Autodesk Inventor part; units mm, degrees
ref_plane "YZ Plane" through (0, 0, 0) normal (1, 0, 0) x (0, 1, 0)
ref_plane "XZ Plane" through (0, 0, 0) normal (0, 1, 0) x (-1, 0, 0)
ref_plane "XY Plane" through (0, 0, 0) normal (0, 0, 1) x (1, 0, 0)
sketch "Sketch1" plane through (0, 0, 0) normal (0, 0, 1) x (1, 0, 0)
  line L0 (-14.25, -14.5) -> (13.65, -14.5)
  line L1 (-13.65, -55.2958) -> (14.25, -55.2958)
  line L2 (50, 0) -> (-50, 0)
  line L3 (-50, 0) -> (-50, -90)
  line L4 (-50, -90) -> (50, -90)
  line L5 (50, -90) -> (50, 0)
  line L6 (50, -86.2958) -> (-50, -86.2958)
  line L7 (14.65, -6.65) -> (-15.25, -6.65)
  line L8 (-15.25, -6.65) -> (-15.25, -22.35)
  line L9 (-15.25, -22.35) -> (14.65, -22.35)
  line L10 (14.65, -22.35) -> (14.65, -6.65)
  line L11 (15.25, -47.4458) -> (-14.65, -47.4458)
  line L12 (-14.65, -47.4458) -> (-14.65, -63.1458)
  line L13 (-14.65, -63.1458) -> (15.25, -63.1458)
  line L14 (15.25, -63.1458) -> (15.25, -47.4458)
  line L15 (30.5, -65.2958) -> (29.35, -65.2958)
  line L16 (-30.5, -65.2958) -> (-29.35, -65.2958)
  circle A0 centre (20.65, -24.0677) radius 2.25
  circle A1 centre (22.6692, -56.1259) radius 2.25
  circle A2 centre (22.25, -13.4966) radius 2.25
  line L17 (19.75, -61.0677) -> (19.75, -50.9236)
  line L18 (19.75, -50.9236) -> (23.15, -50.9236)
  line L19 (23.15, -50.9236) -> (23.15, -46.7261)
  line L20 (19.75, -46.7261) -> (23.15, -46.7261)
  line L21 (19.75, -46.7261) -> (19.75, -44.8549)
  line L22 (19.75, -44.8549) -> (17.65, -44.8549)
  line L23 (17.65, 0) -> (17.65, -44.8549)
  line L24 (17.65, 0) -> (26.85, 0)
  line L25 (26.85, -65.2958) -> (26.85, 0)
  line L26 (23.15, -65.2958) -> (26.85, -65.2958)
  line L27 (23.15, -65.2958) -> (23.15, -61.0677)
  line L28 (19.75, -61.0677) -> (23.15, -61.0677)
  circle A3 centre (-24.3428, -2.5072) radius 2.25
  circle A4 centre (-20.65, -57.8419) radius 2.25
  circle A5 centre (-20.65, -44.9257) radius 2.25
  circle A6 centre (-23.3, -12.9282) radius 2.25
  line L29 (-26.85, 0) -> (-17.65, 0)
  line L30 (-17.65, -4.0591) -> (-17.65, 0)
  line L31 (-19.75, -4.0591) -> (-17.65, -4.0591)
  line L32 (-19.75, -4.7124) -> (-19.75, -4.0591)
  line L33 (-19.75, -4.7124) -> (-23.15, -4.7124)
  line L34 (-23.15, -4.7124) -> (-23.15, -8.7282)
  line L35 (-19.75, -8.7282) -> (-23.15, -8.7282)
  line L36 (-19.75, -18.8723) -> (-19.75, -8.7282)
  line L37 (-19.75, -18.8723) -> (-23.15, -18.8723)
  line L38 (-23.15, -18.8723) -> (-23.15, -23.0697)
  line L39 (-19.75, -23.0697) -> (-23.15, -23.0697)
  line L40 (-19.75, -24.9409) -> (-19.75, -23.0697)
  line L41 (-19.75, -24.9409) -> (-17.65, -24.9409)
  line L42 (-17.65, -65.2958) -> (-17.65, -24.9409)
  line L43 (-26.85, -65.2958) -> (-17.65, -65.2958)
  line L44 (-26.85, 0) -> (-26.85, -65.2958)
  line L45 (-17.65, -4.0591) -> (-17.65, -24.9409)
  line L46 (23.15, -65.2958) -> (17.65, -65.2958)
  line L47 (17.65, -65.2958) -> (17.65, -44.8549)
  line L48 (17.65, -6.65) -> (-17.65, -6.65)
  line L49 (-17.65, -63.1458) -> (17.65, -63.1458)
  line L50 (-26.85, -65.2958) -> (-26.85, -13)
  line L51 (-26.85, -65.2958) -> (-29.35, -65.2958)
  line L52 (-29.35, -65.2958) -> (-29.35, -19)
  line L53 (-29.35, -19) -> (-36.25, -19)
  line L54 (-36.25, -13) -> (-36.25, -19)
  line L55 (-26.85, -13) -> (-36.25, -13)
  line L56 (26.85, -13) -> (26.85, -65.2958)
  line L57 (26.85, -13) -> (36.25, -13)
  line L58 (36.25, -19) -> (36.25, -13)
  line L59 (29.35, -19) -> (36.25, -19)
  line L60 (29.35, -19) -> (29.35, -65.2958)
  line L61 (29.35, -65.2958) -> (26.85, -65.2958)
  line L62 (-26.85, -3) -> (-26.85, 0)
  line L63 (-26.85, -3) -> (-36.25, -3)
  line L64 (-36.25, 0) -> (-36.25, -3)
  line L65 (-26.85, 0) -> (-36.25, 0)
  line L66 (26.85, 0) -> (26.85, -3)
  line L67 (26.85, 0) -> (36.25, 0)
  line L68 (36.25, -3) -> (36.25, 0)
  line L69 (26.85, -3) -> (36.25, -3)
  arc A7 (26.85, -66.2958) -> (29.85, -69.2958) centre (29.85, -66.2958) ccw
  line L70 (26.85, -65.2958) -> (26.85, -66.2958)
  line L71 (26.85, -65.2958) -> (50, -65.2958)
  line L72 (50, -65.2958) -> (50, -85.9433)
  line L73 (34.5, -85.9433) -> (50, -85.9433)
  line L74 (34.5, -78.442) -> (34.5, -85.9433)
  line L75 (34.5, -78.442) -> (45.421, -78.442)
  arc A8 (45.421, -78.442) -> (46.8031, -78.442) centre (46.112, -80.4779) ccw
  line L76 (46.8031, -78.442) -> (49, -78.442)
  line L77 (49, -78.442) -> (49, -69.922)
  line L78 (49, -69.922) -> (46.525, -69.922)
  line L79 (46.525, -69.922) -> (32.6782, -69.3038)
  arc A9 (32.6782, -69.3038) -> (32.5, -69.2958) centre (32.5, -71.2958) ccw
  line L80 (32.5, -69.2958) -> (29.85, -69.2958)
  arc A10 (-29.85, -69.2958) -> (-26.85, -66.2958) centre (-29.85, -66.2958) ccw
  line L81 (-32.5, -69.2958) -> (-29.85, -69.2958)
  arc A11 (-32.5, -69.2958) -> (-32.6782, -69.3038) centre (-32.5, -71.2958) ccw
  line L82 (-32.6782, -69.3038) -> (-46.525, -69.922)
  line L83 (-46.525, -69.922) -> (-49, -69.922)
  line L84 (-49, -69.922) -> (-49, -78.442)
  line L85 (-49, -78.442) -> (-46.8031, -78.442)
  arc A12 (-46.8031, -78.442) -> (-45.421, -78.442) centre (-46.112, -80.4779) ccw
  line L86 (-45.421, -78.442) -> (-34.5, -78.442)
  line L87 (-34.5, -78.442) -> (-34.5, -85.9433)
  line L88 (-34.5, -85.9433) -> (-50, -85.9433)
  line L89 (-50, -65.2958) -> (-50, -85.9433)
  line L90 (-26.85, -65.2958) -> (-50, -65.2958)
  line L91 (-26.85, -65.2958) -> (-26.85, -66.2958)
  line L92 (36.25, 0) -> (36.25, -19)
  line L93 (-36.25, -19) -> (-36.25, 0)
  point P0 (0, 0)
  point P1 (26.95, 0)
  point P2 (-15.25, -6.65)
  dimension "d0" = 50
  dimension "d1" = 50
  dimension "d2" = 90
  dimension "d3" = 7.85
  dimension "d4" = 7.85
  dimension "d5" = 1
  dimension "d6" = 1
  dimension "d7" = 7.85
  dimension "d8" = 7.85
  dimension "d9" = 1
  dimension "d10" = 1
  dimension "d21" = 0
extrude "Extrusion4" add sketch "Sketch1" along normal blind 2 contours L68 L69 L25 L2 | L5 L73 L74 L75 A8 L76 L77 L78 L79 A9 L80 A7 L70 L61 L15 L71 | L92 L57 L25 L69 | L5 L6 L3 L88 L87 L86 A12 L85 L84 L83 L82 A11 L81 A10 L91 L43 L42 L49 L13 L47 L46 L26 L70 A7 L80 A9 L79 L78 L77 L76 A8 L75 L74 L73 | L58 L59 L60 L61 L25 L57 | L44 L63 L64 L2 | L3 L90 L16 L51 L91 A10 L81 A11 L82 L83 L84 L85 A12 L86 L87 L88 | L44 L55 L93 L63 | L44 L51 L52 L53 L54 L55
extrude "Extrusion5" add sketch "Sketch1" against normal blind 0.4 contours L68 L69 L25 L2 | L5 L73 L74 L75 A8 L76 L77 L78 L79 A9 L80 A7 L70 L61 L15 L71 | L25 L26 L27 L28 L17 L18 L19 L20 L21 L22 L23 L2 | L92 L57 L25 L69 | L5 L6 L3 L88 L87 L86 A12 L85 L84 L83 L82 A11 L81 A10 L91 L43 L42 L49 L13 L47 L46 L26 L70 A7 L80 A9 L79 L78 L77 L76 A8 L75 L74 L73 | L23 L48 L7 L45 L30 L2 | L58 L59 L60 L61 L25 L57 | L30 L31 L32 L33 L34 L35 L36 L37 L38 L39 L40 L41 L42 L43 L44 L2 | L23 L47 L49 L14 L11 L12 L42 L45 L48 L8 L9 L10 | L44 L63 L64 L2 | L45 L41 L40 L39 L38 L37 L36 L35 L34 L33 L32 L31 | L22 L21 L20 L19 L18 L17 L28 L27 L46 L47 | L10 L9 L8 L7 | L3 L90 L16 L51 L91 A10 L81 A11 L82 L83 L84 L85 A12 L86 L87 L88 | L44 L55 L93 L63 | L44 L51 L52 L53 L54 L55 | L13 L12 L11 L14 | A0 | A1 | A2 | A3 | A4 | A5 | A6
sketch "Sketch2" plane through (50, -86.2958, 2) normal (1, 0, 0) x (0, 0, -1)
  line L0 (2.2133, 0.4205) -> (-23.8, -4.5217)
  line L1 (-23.8, -4.5217) -> (-23.6133, -5.5042)
  line L2 (-23.6133, -5.5042) -> (2.4, -0.5619)
  line L3 (2.4, -0.5619) -> (2.2133, 0.4205)
  line L4 (0, -10.5619) -> (0, 0.2036)
  line L5 (0, 0.2036) -> (2.4, 0.6596)
  line L6 (2.4, 0.6596) -> (2.4, -10.5619)
  line L7 (2.4, -10.5619) -> (0, -10.5619)
  point P0 (2, 86.2958)
  dimension "d15" = 2.4
  dimension "d16" = 0.2
  dimension "d17" = 0
  dimension "d18" = 10
extrude "Extrusion3" cut sketch "Sketch2" against normal through all contours L3 L2 L4 L0 | L0 L4 L5 L6 L3 | L6 L7 L4 L2
sketch "Sketch3" plane through (0, 0, -0.4) normal (0, 0, -1) x (-1, 0, 0)
  circle A0 centre (24.3428, -2.5072) radius 1.5
  circle A1 centre (23.3, -12.9282) radius 1.5
  circle A2 centre (20.65, -58.1775) radius 1.5
  circle A3 centre (20.65, -45.2613) radius 1.5
  circle A4 centre (-20.65, -23.7673) radius 1.5
  circle A5 centre (-22.25, -55.8509) radius 1.5
  circle A6 centre (-22.253, -13.1962) radius 1.5
  arc A7 (-26.256, -0.1) -> (-26.756, -0.6) centre (-26.256, -0.6) ccw
  line L0 (-26.756, -0.6) -> (-26.756, -64.6958)
  arc A8 (-26.756, -64.6958) -> (-26.256, -65.1958) centre (-26.256, -64.6958) ccw
  line L1 (-26.256, -65.1958) -> (-23.756, -65.1958)
  arc A9 (-23.756, -65.1958) -> (-23.256, -64.6958) centre (-23.756, -64.6958) ccw
  line L2 (-23.256, -64.6958) -> (-23.256, -61.4677)
  arc A10 (-22.756, -60.9677) -> (-23.256, -61.4677) centre (-22.756, -61.4677) ccw
  line L3 (-22.756, -60.9677) -> (-20.35, -60.9677)
  arc A11 (-20.35, -60.9677) -> (-19.85, -60.4677) centre (-20.35, -60.4677) ccw
  line L4 (-19.85, -60.4677) -> (-19.85, -51.8592)
  arc A12 (-19.85, -51.8592) -> (-20.35, -51.3592) centre (-20.35, -51.8592) ccw
  line L5 (-20.35, -51.3592) -> (-22.756, -51.3592)
  arc A13 (-23.256, -50.8592) -> (-22.756, -51.3592) centre (-22.756, -50.8592) ccw
  line L6 (-23.256, -50.8592) -> (-23.256, -41.5958)
  arc A14 (-22.756, -41.0958) -> (-23.256, -41.5958) centre (-22.756, -41.5958) ccw
  line L7 (-22.756, -41.0958) -> (-12.25, -41.0958)
  arc A15 (-11.75, -41.5958) -> (-12.25, -41.0958) centre (-12.25, -41.5958) ccw
  line L8 (-11.75, -41.5958) -> (-11.75, -43.0958)
  arc A16 (-11.75, -43.0958) -> (-11.25, -43.5958) centre (-11.25, -43.0958) ccw
  line L9 (-11.25, -43.5958) -> (11.25, -43.5958)
  arc A17 (11.25, -43.5958) -> (11.75, -43.0958) centre (11.25, -43.0958) ccw
  line L10 (11.75, -43.0958) -> (11.75, -41.5958)
  arc A18 (12.25, -41.0958) -> (11.75, -41.5958) centre (12.25, -41.5958) ccw
  line L11 (12.25, -41.0958) -> (17.25, -41.0958)
  arc A19 (17.75, -41.5958) -> (17.25, -41.0958) centre (17.25, -41.5958) ccw
  line L12 (17.75, -41.5958) -> (17.75, -64.6958)
  arc A20 (17.75, -64.6958) -> (18.25, -65.1958) centre (18.25, -64.6958) ccw
  line L13 (18.25, -65.1958) -> (26.25, -65.1958)
  arc A21 (26.25, -65.1958) -> (26.75, -64.6958) centre (26.25, -64.6958) ccw
  line L14 (26.75, -64.6958) -> (26.75, -0.6)
  arc A22 (26.75, -0.6) -> (26.25, -0.1) centre (26.25, -0.6) ccw
  line L15 (26.25, -0.1) -> (18.25, -0.1)
  arc A23 (18.25, -0.1) -> (17.75, -0.6) centre (18.25, -0.6) ccw
  line L16 (17.75, -0.6) -> (17.75, -3.1235)
  arc A24 (17.75, -3.1235) -> (18.25, -3.6235) centre (18.25, -3.1235) ccw
  line L17 (18.25, -3.6235) -> (22.75, -3.6235)
  arc A25 (23.25, -4.1235) -> (22.75, -3.6235) centre (22.75, -4.1235) ccw
  line L18 (23.25, -4.1235) -> (23.25, -8.3282)
  arc A26 (22.75, -8.8282) -> (23.25, -8.3282) centre (22.75, -8.3282) ccw
  line L19 (22.75, -8.8282) -> (20.35, -8.8282)
  arc A27 (20.35, -8.8282) -> (19.85, -9.3282) centre (20.35, -9.3282) ccw
  line L20 (19.85, -9.3282) -> (19.85, -17.9366)
  arc A28 (19.85, -17.9366) -> (20.35, -18.4366) centre (20.35, -17.9366) ccw
  line L21 (20.35, -18.4366) -> (22.75, -18.4366)
  arc A29 (23.25, -18.9366) -> (22.75, -18.4366) centre (22.75, -18.9366) ccw
  line L22 (23.25, -18.9366) -> (23.25, -28.2)
  arc A30 (22.75, -28.7) -> (23.25, -28.2) centre (22.75, -28.2) ccw
  line L23 (22.75, -28.7) -> (12.25, -28.7)
  arc A31 (11.75, -28.2) -> (12.25, -28.7) centre (12.25, -28.2) ccw
  line L24 (11.75, -28.2) -> (11.75, -26.7)
  arc A32 (11.75, -26.7) -> (11.25, -26.2) centre (11.25, -26.7) ccw
  line L25 (11.25, -26.2) -> (-17.25, -26.2)
  arc A33 (-17.75, -25.7) -> (-17.25, -26.2) centre (-17.25, -25.7) ccw
  line L26 (-17.75, -25.7) -> (-17.75, -0.6)
  arc A34 (-17.75, -0.6) -> (-18.25, -0.1) centre (-18.25, -0.6) ccw
  line L27 (-18.25, -0.1) -> (-26.256, -0.1)
  line L28 (-29.5, -65.8371) -> (-50, -65.8371)
  line L29 (-50, -65.8371) -> (-50, -86.3723)
  line L30 (-34.5, -86.3723) -> (-50, -86.3723)
  line L31 (-34.5, -78.883) -> (-34.5, -86.3723)
  line L32 (-34.5, -78.883) -> (-49, -78.883)
  line L33 (-49, -70.278) -> (-33.7527, -70.278)
  line L34 (-32.5, -69.8371) -> (-31.5, -69.8371)
  line L35 (29.5, -65.8371) -> (50, -65.8371)
  line L36 (33.7527, -70.278) -> (49, -70.278)
  line L37 (49, -78.883) -> (34.5, -78.883)
  circle A35 centre (-47.662, -81.0191) radius 2.15
  circle A36 centre (-46.75, -81.383) radius 1.5
  line L38 (34.5, -78.883) -> (34.5, -86.3723)
  line L39 (29.5, -67.8371) -> (29.5, -65.8371)
  arc A37 (29.5, -67.8371) -> (31.5, -69.8371) centre (31.5, -67.8371) ccw
  line L40 (32.5, -69.8371) -> (31.5, -69.8371)
  arc A38 (33.7527, -70.278) -> (32.5, -69.8371) centre (32.5, -71.8371) ccw
  arc A39 (-31.5, -69.8371) -> (-29.5, -67.8371) centre (-31.5, -67.8371) ccw
  line L41 (-29.5, -67.8371) -> (-29.5, -65.8371)
  arc A40 (-32.5, -69.8371) -> (-33.7527, -70.278) centre (-32.5, -71.8371) ccw
  line L42 (-49, -78.883) -> (-49, -70.278)
  line L43 (49, -70.278) -> (49, -78.883)
  line L44 (34.5, -86.3723) -> (50, -86.3723)
  line L45 (50, -65.8371) -> (50, -86.3723)
  circle A41 centre (46.75, -81.383) radius 1.5
  point P0 (0, 0)
  point P1 (-49, -78.442)
  point P2 (-49, -78.292)
  point P3 (-50, -86.5495)
  point P4 (-34.5, -86.5495)
  point P5 (-50, -66.2871)
  point P6 (-34.5, -78.8554)
  point P7 (-49, -70.3354)
  point P8 (49, -78.2054)
  point P9 (49, -77.792)
  point P10 (36.05, -86.3723)
hole "Hole1" at (22.25, -55.8509, -0.4) at (20.65, -23.7673, -0.4) at (22.253, -13.1962, -0.4) at (-24.3428, -2.5072, -0.4) at (-23.3, -12.9282, -0.4) at (-20.65, -45.2613, -0.4) at (-20.65, -58.1775, -0.4) direction (0, 0, 1) diameter 3.4 depth 10 countersink diameter 6 countersink angle 90
equation "\"d4\" = d3"
equation "\"d6\" = d5"
equation "\"d7\" = d3"
equation "\"d8\" = d3"
equation "\"d9\" = d5"
equation "\"d10\" = d5"
properties part number "Ceiling"
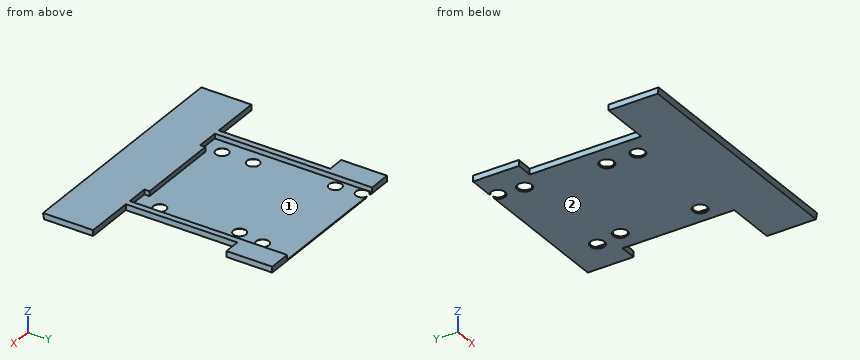
Check sheet for the modelled part. Datum: model origin and axes. Units: mm. Face numbers are marked on the shaded views. Round coordinates to 2 decimals unless told otherwise and drop trailing zeros. Loops run counter-clockwise (first coordinate to the right, second up) from the corner with the lowest first, then second, coordinate; pieces in that order, holes last. Notation, with made-up numbers: M -33,38 L -19,38 A23 cw -19,77 Z; hole C 13,-0.5 d6. An arc over 180 degrees is marked long. Answer as a JSON object with one key per item and string values.
1. Section check B-B (z = 0.65). Record the boundary of the cut face in (x, y), plus the area to 3 significant figures.
Reply:
{"outline": "M -50,-85.84 L 50,-85.84 L 50,-65.3 L 29.35,-65.3 L 29.35,-19 L 36.25,-19 L 36.25,0 L 26.85,0 L 26.85,-65.3 L 17.65,-65.3 L 17.65,-63.15 L -17.65,-63.15 L -17.65,-65.3 L -26.85,-65.3 L -26.85,0 L -36.25,0 L -36.25,-19 L -29.35,-19 L -29.35,-65.3 L -50,-65.3 Z", "area": "2,720 mm²"}
2. Mould release check, pull along X, two halves, no side actions. Record for the marked faces 1 and 2: pulls with the +X half, pulls with the -X half, needs draft (parallel to the pull), parting line crosses it, or undercut.
Reply:
{"face 1": "undercut", "face 2": "needs draft"}
3. Scan lines: line 1 (X direction, y = -53.5, z = 0.45); line 2 (X direction, y = -6, z = 1.2); line 3 (Y direction, x = -34.5, z = 1.15). Record each from-to range of solid material in increasing order.
Reply:
{"line 1": "x = -29.35 to -26.85, 26.85 to 29.35", "line 2": "x = -36.25 to -26.85, 26.85 to 36.25", "line 3": "y = -85.93 to -65.3, -19 to 0"}
4. Gauge pin test, flat ends, axial feed: P1, Ø1, axis at y = -21.5, z = 1, coming from the +X side; P2, Ø0.7, axis at y = -40, z = 0.5, coming from the -X side; P3, Ø1, axis at y = -18, z = 0.5, coming from the -X side. Record the tip position at first contact, or that the pin passes through.
Reply:
{"P1": "stops at x = 29.35", "P2": "stops at x = -29.35", "P3": "stops at x = -36.25"}
5. Section check A-A (x = -35). Record the boundary of the cut face in (y, z).
Reply:
{"outline": "M -86.09,2 L -85.64,-0.4 L -65.3,-0.4 L -65.3,2 Z; M -19,-0.4 L 0,-0.4 L 0,2 L -19,2 Z"}
6. Section check C-C (x = 20.65). State how many separate pieces and enclosed holes the cut face has, plus the area to 3 significant figures.
Reply:
{"separate pieces": "4", "enclosed holes": "0", "area": "69.6 mm²"}
